Drawing for the job (mm, zero at the part's lowest x, y, z). Give positions to 0.01 mm unless a question says otherwise; leave off trailing zeros. Order: outer loops, then holes, each group sorted by start corner. A loop starts at its lowest first (then second) coordinate and runs counter-clockwise, first axis right, second up. Notation, with made-up numbers: M -27.5,-32.5 L 25.5,-32.5 A13 ccw 25.5,-18.5 Z; hole C 11,-24.5 d11. An arc over 180 degrees is marked long. One line per item, written item: value.
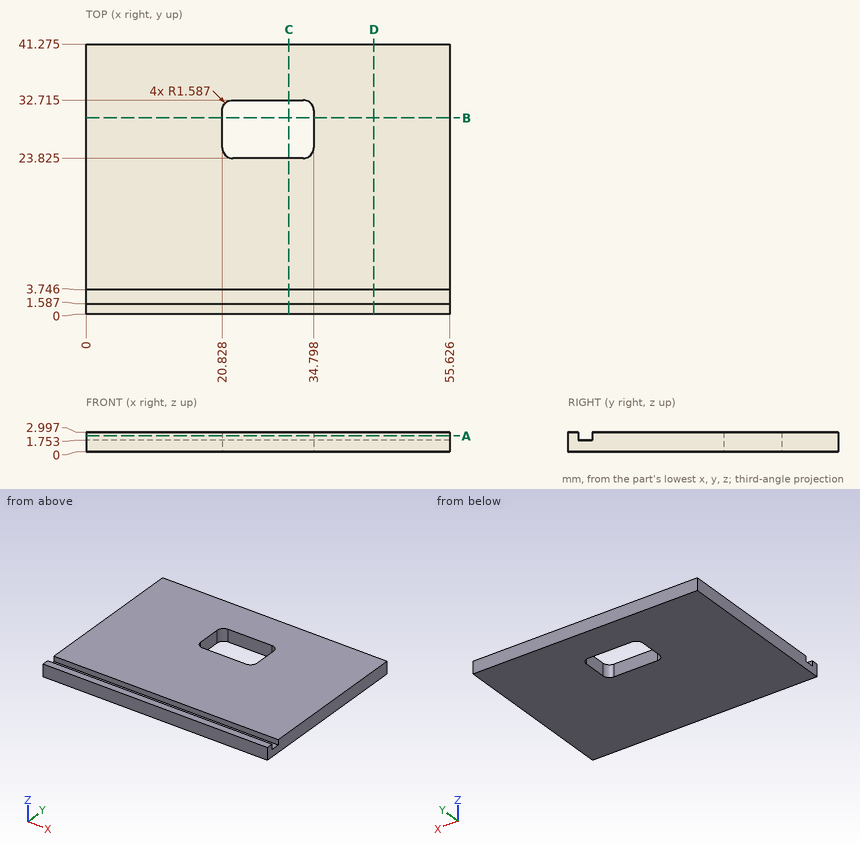
1) Pin check, flat tip, straight feed: pin 1 (4 mm diameter, centred on x = 39, y = 22, fed in from -Z). Stop position of the tip, or through.
Check values:
pin 1: z = 0
2) Saw through at A-A, the plane z = 2.4. Write the cut outline in (x, y) (1 decimal), then the cut area to 3 significant figures.
Check values:
outline: M 0,0 L 55.6,0 L 55.6,1.6 L 0,1.6 Z; M 0,3.7 L 55.6,3.7 L 55.6,41.3 L 0,41.3 Z; hole M 20.8,25.4 A1.6 ccw 22.4,23.8 L 33.2,23.8 A1.6 ccw 34.8,25.4 L 34.8,31.1 A1.6 ccw 33.2,32.7 L 22.4,32.7 A1.6 ccw 20.8,31.1 Z
area: 2,050 mm^2
3) Saw through at B-B, the plane y = 30. Write the cut outline in (x, z) (1 decimal), then the cut area to 3 significant figures.
Check values:
outline: M 0,0 L 20.8,0 L 20.8,3 L 0,3 Z; M 34.8,0 L 55.6,0 L 55.6,3 L 34.8,3 Z
area: 125 mm^2
4) Saw through at C-C, the plane x = 31. Write the cut outline in (y, z) (1 decimal).
Check values:
outline: M 0,0 L 23.8,0 L 23.8,3 L 3.7,3 L 3.7,1.8 L 1.6,1.8 L 1.6,3 L 0,3 Z; M 32.7,0 L 41.3,0 L 41.3,3 L 32.7,3 Z
5) Saw through at D-D, the plane x = 44. Write the cut outline in (y, z) (1 decimal), then the cut area to 3 significant figures.
Check values:
outline: M 0,0 L 41.3,0 L 41.3,3 L 3.7,3 L 3.7,1.8 L 1.6,1.8 L 1.6,3 L 0,3 Z
area: 121 mm^2
6) Drill centre lines: probe 1 along Y at (x, z) = (20, 2.65) (1 decimal); probe 2 along Y at (x, z) = (25.5, 1.2) (1 decimal); probe 3 along X at (y, z) = (25, 1.05) (1 decimal). Where is each one in solid material? Low to high. Write a range as from..to.
Check values:
probe 1: 0..1.6, 3.7..41.3
probe 2: 0..23.8, 32.7..41.3
probe 3: 0..20.9, 34.7..55.6
